Autodesk Fusion 360 part; units mm, degrees
sketch "Skizze1" plane through (0, 0, 0) normal (0, 0, 1) x (1, 0, 0)
  line L0 (0, 0) -> (60, 0)
  line L1 (60, 0) -> (60, 140)
  line L2 (60, 140) -> (0, 140)
  line L3 (0, 140) -> (0, 0)
  dimension "d1" = 60
  dimension "d2" = 140
extrude "Extrusion1" add sketch "Skizze1" along normal blind 20
sketch "Skizze2" plane through (60, 0, 0) normal (1, 0, 0) x (0, 1, 0)
  line L0 (0, 0) -> (140, 0)
  line L1 (140, 0) -> (140, 20)
  line L2 (140, 20) -> (0, 20)
  line L3 (0, 20) -> (0, 0)
  circle A0 centre (30, 10) radius 4.15
  circle A1 centre (100.3, 10) radius 4.15
  point P0 (0, 10)
  dimension "d5" = 8.3
  dimension "d6" = 8.3
extrude "Extrusion2" cut sketch "Skizze2" against normal blind 50 contours A0 | A1
sketch "Skizze3" plane through (0, 0, 20) normal (0, 0, 1) x (-1, 0, 0)
  line L0 (0, -140) -> (0, 0)
  line L1 (0, 0) -> (-60, 0)
  line L2 (-60, 0) -> (-60, -140)
  line L3 (-60, -140) -> (0, -140)
  circle A0 centre (-31.6, -24.1) radius 1.7
  circle A1 centre (-7.7, -24.1) radius 1.7
  circle A2 centre (-31.6, -6.2) radius 1.7
  circle A3 centre (-7.7, -6.2) radius 1.7
  circle A4 centre (-7.7, -107.4) radius 1.7
  circle A5 centre (-31.6, -125.3) radius 1.7
  circle A6 centre (-7.7, -125.3) radius 1.7
  circle A7 centre (-31.6, -107.4) radius 1.7
  dimension "d9" = 3.4
  dimension "d10" = 3.4
  dimension "d11" = 3.4
  dimension "d12" = 3.4
  dimension "d13" = 3.4
  dimension "d14" = 3.4
  dimension "d15" = 3.4
  dimension "d16" = 3.4
extrude "Extrusion3" cut sketch "Skizze3" against normal blind 20 contours A0 | A1 | A2 | A3 | A4 | A5 | A6 | A7
sketch "Skizze5" plane through (0, 0, 0) normal (0, 0, -1) x (1, 0, 0)
  line L0 (0, 0) -> (0, -140)
  line L1 (0, -140) -> (60, -140)
  line L2 (60, -140) -> (60, 0)
  line L3 (60, 0) -> (0, 0)
  circle A0 centre (46, -130) radius 1
  circle A1 centre (7.7, -125.3) radius 1.7
  circle A2 centre (31.6, -24.1) radius 1.7
  circle A3 centre (31.6, -6.2) radius 1.7
  circle A4 centre (31.6, -125.3) radius 1.7
  circle A5 centre (7.7, -107.4) radius 1.7
  circle A6 centre (7.7, -24.1) radius 1.7
  circle A7 centre (7.7, -6.2) radius 1.7
  circle A8 centre (31.6, -107.4) radius 1.7
  dimension "d22" = 2
sketch "Skizze6" plane through (0, 0, 0) normal (0, 0, -1) x (1, 0, 0)
  circle A0 centre (7.7, -125.3) radius 1.7
  circle A1 centre (31.6, -24.1) radius 1.7
  circle A2 centre (31.6, -6.2) radius 1.7
  circle A3 centre (31.6, -125.3) radius 1.7
  circle A4 centre (7.7, -107.4) radius 1.7
  circle A5 centre (7.7, -24.1) radius 1.7
  circle A6 centre (7.7, -6.2) radius 1.7
  circle A7 centre (31.6, -107.4) radius 1.7
  line L0 (0, 0) -> (0, -140)
  line L1 (0, -140) -> (60, -140)
  line L2 (60, -140) -> (60, 0)
  line L3 (60, 0) -> (0, 0)
  line L4 (60, -53.1468) -> (40, -53.1468)
  line L5 (40, -53.1468) -> (40, -85.1468)
  line L6 (40, -85.1468) -> (60, -85.1468)
  line L7 (60, -85.1468) -> (60, -53.1468)
  line L8 (60, -53.1468) -> (40, -53.1468)
  line L9 (40, -53.1468) -> (40, -58.1468)
  line L10 (40, -58.1468) -> (60, -58.1468)
  line L11 (60, -58.1468) -> (60, -53.1468)
  line L12 (40, -85.1468) -> (60, -85.1468)
  line L13 (60, -85.1468) -> (60, -80.1468)
  line L14 (60, -80.1468) -> (40, -80.1468)
  line L15 (40, -80.1468) -> (40, -85.1468)
  line L16 (53.5, -63.5) -> (36.5, -63.5)
  arc A8 (36.5, -63.5) -> (36.5, -66.5) centre (36.5, -65) ccw
  line L17 (36.5, -66.5) -> (53.5, -66.5)
  arc A9 (53.5, -66.5) -> (53.5, -63.5) centre (53.5, -65) ccw
  line L18 (55, -65) -> (35, -65) construction
  line L19 (36.5, -75.4708) -> (53.5, -75.4708)
  arc A10 (53.5, -75.4708) -> (53.5, -72.4708) centre (53.5, -73.9708) ccw
  line L20 (53.5, -72.4708) -> (36.5, -72.4708)
  arc A11 (36.5, -72.4708) -> (36.5, -75.4708) centre (36.5, -73.9708) ccw
  line L21 (35, -73.9708) -> (55, -73.9708) construction
  dimension "d31" = 20
  dimension "d32" = 32
  dimension "d33" = 20
  dimension "d34" = 5
  dimension "d35" = 20
  dimension "d36" = 5
  dimension "d72" = 3
  dimension "d73" = 3
extrude "Extrusion19" cut sketch "Skizze6" against normal blind 1 contours L5 L16 L17 A9 | L5 L16 A8 L17 | L5 L19 L20 A11 | L5 L19 A10 L20
extrude "Extrusion7" add sketch "Skizze6" along normal blind 12 contours L2 L4 L5 L7 L8 L9 L10 L11 | L2 L5 L6 L7 L12 L13 L14 L15
sketch "Skizze8" plane through (0, 0, 0) normal (-1, 0, 0) x (0, -1, 0)
  line L0 (-140, 0) -> (0, 0)
  line L1 (0, 0) -> (0, 20)
  line L2 (0, 20) -> (-140, 20)
  line L3 (-140, 20) -> (-140, 0)
  circle A0 centre (-15, 10) radius 2.2
  circle A1 centre (-45, 10) radius 2.2
  dimension "d27" = 4.4
  dimension "d28" = 4.4
extrude "Extrusion6" cut sketch "Skizze8" against normal blind 60 contours A0 | A1
sketch "Skizze10" plane through (60, 0, 0) normal (1, 0, 0) x (0, 1, 0)
  line L0 (58.1468, -12) -> (58.1468, 0)
  line L1 (58.1468, 0) -> (80.1468, 0)
  line L2 (80.1468, 0) -> (80.1468, -12)
  circle A0 centre (15, 10) radius 2.2
  circle A1 centre (45, 10) radius 2.2
  circle A2 centre (30, 10) radius 4.15
  circle A3 centre (100.3, 10) radius 4.15
  line L3 (53.1468, -12) -> (58.1468, -12)
  line L4 (85.1468, -12) -> (85.1468, 0)
  line L5 (85.1468, 0) -> (140, 0)
  line L6 (140, 0) -> (140, 20)
  line L7 (140, 20) -> (0, 20)
  line L8 (0, 20) -> (0, 0)
  line L9 (0, 0) -> (53.1468, 0)
  line L10 (53.1468, 0) -> (53.1468, -12)
  circle A4 centre (15, 10) radius 7.5
  circle A5 centre (45, 10) radius 7.5
  line L11 (80.1468, -12) -> (85.1468, -12)
  dimension "d42" = 15
  dimension "d43" = 15
extrude "Extrusion9" cut sketch "Skizze10" against normal blind 10 contours A4 | A5
sketch "Skizze13" plane through (0, 0, 20) normal (0, 0, 1) x (-1, 0, 0)
  circle A0 centre (-7.7, -125.3) radius 1.7
  circle A1 centre (-31.6, -24.1) radius 1.7
  circle A2 centre (-31.6, -6.2) radius 1.7
  circle A3 centre (-31.6, -125.3) radius 1.7
  circle A4 centre (-7.7, -107.4) radius 1.7
  circle A5 centre (-7.7, -24.1) radius 1.7
  circle A6 centre (-7.7, -6.2) radius 1.7
  circle A7 centre (-31.6, -107.4) radius 1.7
  line L0 (0, -140) -> (0, 0)
  line L1 (0, 0) -> (-60, 0)
  line L2 (-60, 0) -> (-60, -140)
  line L3 (-60, -140) -> (0, -140)
  circle A8 centre (-47, -10) radius 7.5
  dimension "d53" = 15
extrude "Extrusion12" cut sketch "Skizze13" against normal blind 5 contours A8
sketch "Skizze14" plane through (0, 0, 15) normal (0, 0, 1) x (-1, 0, 0)
  line L0 (-50, -9.4098) -> (-50, -16.8739)
  arc A0 (-50, -16.8739) -> (-54.4767, -9.4098) centre (-47, -10) ccw
  line L1 (-54.4767, -9.4098) -> (-50, -9.4098)
  circle A1 centre (-47, -10) radius 1
  dimension "d56" = 2
extrude "Extrusion13" cut sketch "Skizze14" against normal blind 1 contours A1
sketch "Skizze15" plane through (0, 0, 20) normal (0, 0, 1) x (-1, 0, 0)
  circle A0 centre (-47, -10) radius 7.5
  circle A1 centre (-7.7, -125.3) radius 1.7
  circle A2 centre (-31.6, -24.1) radius 1.7
  circle A3 centre (-31.6, -6.2) radius 1.7
  circle A4 centre (-31.6, -125.3) radius 1.7
  circle A5 centre (-7.7, -107.4) radius 1.7
  circle A6 centre (-7.7, -24.1) radius 1.7
  circle A7 centre (-7.7, -6.2) radius 1.7
  circle A8 centre (-31.6, -107.4) radius 1.7
  line L0 (0, -140) -> (0, 0)
  line L1 (0, 0) -> (-60, 0)
  line L2 (-60, 0) -> (-60, -140)
  line L3 (-60, -140) -> (0, -140)
  line L4 (-39.5, 0) -> (-54.5, 0)
  line L5 (-54.5, 0) -> (-54.5, -17.5)
  line L6 (-54.5, -17.5) -> (-39.5, -17.5)
  line L7 (-39.5, -17.5) -> (-39.5, 0)
extrude "Extrusion14" cut sketch "Skizze15" against normal blind 7 contours A0 | A0 L1 L4 L5 L7
sketch "Skizze16" plane through (0, 0, 20) normal (0, 0, 1) x (-1, 0, 0)
  circle A0 centre (-31.6, -107.4) radius 1.7
  circle A1 centre (-7.7, -6.2) radius 1.7
  circle A2 centre (-7.7, -24.1) radius 1.7
  circle A3 centre (-7.7, -107.4) radius 1.7
  circle A4 centre (-31.6, -125.3) radius 1.7
  circle A5 centre (-31.6, -6.2) radius 1.7
  circle A6 centre (-31.6, -24.1) radius 1.7
  circle A7 centre (-7.7, -125.3) radius 1.7
  line L0 (-39.5, 0) -> (-39.5, -10)
  arc A8 (-54.5, -10) -> (-39.5, -10) centre (-47, -10) ccw
  line L1 (-54.5, -10) -> (-54.5, 0)
  line L2 (-54.5, 0) -> (-60, 0)
  line L3 (-60, 0) -> (-60, -140)
  line L4 (-60, -140) -> (0, -140)
  line L5 (0, -140) -> (0, 0)
  line L6 (0, 0) -> (-39.5, 0)
  circle A9 centre (-46, -130) radius 7.5
  line L7 (-38.5, -140) -> (-53.5, -140)
  line L8 (-53.5, -140) -> (-53.5, -122.5)
  line L9 (-53.5, -122.5) -> (-38.5, -122.5)
  line L10 (-38.5, -122.5) -> (-38.5, -140)
  dimension "d61" = 15
extrude "Extrusion15" cut sketch "Skizze16" against normal blind 7 contours L4 A9 L7 L8 L10 | A9
sketch "Skizze17" plane through (0, 0, 20) normal (0, 0, 1) x (-1, 0, 0)
  line L0 (-38.5, -130) -> (-38.5, -140)
  line L1 (-38.5, -140) -> (0, -140)
  line L2 (0, -140) -> (0, 0)
  line L3 (0, 0) -> (-39.5, 0)
  line L4 (-39.5, 0) -> (-39.5, -10)
  arc A0 (-54.5, -10) -> (-39.5, -10) centre (-47, -10) ccw
  line L5 (-54.5, -10) -> (-54.5, 0)
  line L6 (-54.5, 0) -> (-60, 0)
  line L7 (-60, 0) -> (-60, -140)
  line L8 (-60, -140) -> (-53.5, -140)
  line L9 (-53.5, -140) -> (-53.5, -130)
  arc A1 (-38.5, -130) -> (-53.5, -130) centre (-46, -130) ccw
  circle A2 centre (-31.6, -107.4) radius 1.7
  circle A3 centre (-7.7, -6.2) radius 1.7
  circle A4 centre (-7.7, -24.1) radius 1.7
  circle A5 centre (-7.7, -107.4) radius 1.7
  circle A6 centre (-31.6, -125.3) radius 1.7
  circle A7 centre (-31.6, -6.2) radius 1.7
  circle A8 centre (-31.6, -24.1) radius 1.7
  circle A9 centre (-7.7, -125.3) radius 1.7
  line L10 (-49.25, -92.5) -> (-42.75, -92.5)
  line L11 (-42.75, -92.5) -> (-42.75, -152.5)
  line L12 (-42.75, -152.5) -> (-49.25, -152.5)
  line L13 (-49.25, -152.5) -> (-49.25, -92.5)
  line L14 (-49.25, -92.5) -> (-42.75, -152.5) construction
  line L15 (-42.75, -92.5) -> (-49.25, -152.5) construction
  point P0 (-46, -122.5)
  dimension "d64" = 60
  dimension "d65" = 6.5
extrude "Extrusion16" cut sketch "Skizze17" against normal blind 5 contours A1 L10 L11 L13
sketch "Skizze18" plane through (0, 0, 20) normal (0, 0, 1) x (-1, 0, 0)
  line L0 (-42.75, -92.5) -> (-42.75, -123.2407)
  arc A0 (-38.5, -130) -> (-42.75, -123.2407) centre (-46, -130) ccw
  line L1 (-38.5, -130) -> (-38.5, -140)
  line L2 (-38.5, -140) -> (0, -140)
  line L3 (0, -140) -> (0, 0)
  line L4 (0, 0) -> (-39.5, 0)
  line L5 (-39.5, 0) -> (-39.5, -10)
  arc A1 (-54.5, -10) -> (-39.5, -10) centre (-47, -10) ccw
  line L6 (-54.5, -10) -> (-54.5, 0)
  line L7 (-54.5, 0) -> (-60, 0)
  line L8 (-60, 0) -> (-60, -140)
  line L9 (-60, -140) -> (-53.5, -140)
  line L10 (-53.5, -140) -> (-53.5, -130)
  arc A2 (-49.25, -123.2407) -> (-53.5, -130) centre (-46, -130) ccw
  line L11 (-49.25, -123.2407) -> (-49.25, -92.5)
  line L12 (-49.25, -92.5) -> (-42.75, -92.5)
  circle A3 centre (-31.6, -107.4) radius 1.7
  circle A4 centre (-7.7, -6.2) radius 1.7
  circle A5 centre (-7.7, -24.1) radius 1.7
  circle A6 centre (-7.7, -107.4) radius 1.7
  circle A7 centre (-31.6, -125.3) radius 1.7
  circle A8 centre (-31.6, -6.2) radius 1.7
  circle A9 centre (-31.6, -24.1) radius 1.7
  circle A10 centre (-7.7, -125.3) radius 1.7
  line L13 (-50.25, -47.5) -> (-43.75, -47.5)
  line L14 (-43.75, -47.5) -> (-43.75, 12.5)
  line L15 (-43.75, 12.5) -> (-50.25, 12.5)
  line L16 (-50.25, 12.5) -> (-50.25, -47.5)
  line L17 (-50.25, -47.5) -> (-43.75, 12.5) construction
  line L18 (-43.75, -47.5) -> (-50.25, 12.5) construction
  point P0 (-47, -17.5)
  dimension "d68" = 6.5
  dimension "d69" = 60
extrude "Extrusion17" cut sketch "Skizze18" against normal blind 5 contours A1 L13 L14 L16
extrude "Extrusion18" cut 2 faces at (46.6667, 54.8135, -12) (53.3333, 83.4802, -12) along direction (0, 0, 1) blind 12
CAD build for the part. Positions are in the model's coordinates, mm. A direction names the side the tool comes from. Coordinates: 2 decimals unless noted, no trailing zeros. Write each loop counter-clockwise with the first axis right and the second up, starting at its lowest first coordinate (ties: lowest second). Pieces come first, ordered by that corner, then holes.
(1) Cut at B-B, the plane y = 6.2. List the corners of the cut face in (x, z).
(2) Cut at A-A, the plane x = 31.6. Count the separate pieces of the cut face and the enclosed holes in it, and give its area (3 significant figures).
(3) Cut at C-C, the plane x = 19. List the corners of the cut face in (y, z).
(4) Drill centre lines: probe 1 along Y at (x, z) = (31.6, 15); probe 2 along Y at (x, z) = (47, 10.5); probe 3 along Z at (x, y) = (48, 30). Where is each one in solid material? Low to high.
(5) Two-plate mould, pull along Y, no slides. Class faces 6 (the face through (38.5, 135, 17)), 7 (the face through (50, 47, 8)), 8 (the face through (41.693, 15.3, 15.771)), 9 (the face through (10, 30, 10)): +Y half, -Y half, draft (parallel to the pull), parting line (faces both ways), or undercut.
(6) 3-axis set-ups, long thin cutter, end or side, ignore diameter. For faces 1 (the face through (54.5, 5, 17)), 2 (the face through (10, 100, 10)), 3 (the face through (30.8, 25.6, 10.1)), 4 (the face through (53.5, 135, 17)), 5 (the face through (45, 65, 1)): which of +Z, -Z, +X, -X, +Y, -Y reach the whole face in a straight line?
(7) Flat gauge pins, fed straight in: pin 1 (4 mm diameter, centred on x = 46, z = 17.5, fed in from -Y); pin 2 (7.5 mm diameter, centred on x = 43.5, y = 129, fed in from +Z). Where does each tip first touch, or does it go through?
Geometry says:
1. outline: (0, 0) - (6, 0) - (6, 20) - (0, 20) - close; (9.4, 0) - (29.9, 0) - (29.9, 20) - (9.4, 20) - close; (33.3, 0) - (60, 0) - (60, 20) - (54.5, 20) - (54.5, 13) - (39.5, 13) - (39.5, 20) - (33.3, 20) - close
2. separate pieces: 5
2. enclosed holes: 4
2. area: 2,390 mm2
3. outline: (0, 0) - (140, 0) - (140, 20) - (0, 20) - close; hole circle Ø4.4 at (15, 10); hole circle Ø8.3 at (30, 10); hole circle Ø4.4 at (45, 10); hole circle Ø8.3 at (100.3, 10)
4. probe 1: y = 0 to 4.5, 7.9 to 22.4, 25.8 to 105.7, 109.1 to 123.6, 127 to 140
4. probe 2: y = 0 to 12.86, 17.14 to 25.88, 34.12 to 42.86, 47.14 to 96.18, 104.42 to 140
4. probe 3: z = 0 to 5.85, 14.15 to 15
5. face 6: draft
5. face 7: undercut
5. face 8: -Y half
5. face 9: undercut
6. face 1: +Z, -Y
6. face 2: +X
6. face 3: +Z, -Z
6. face 4: +Z, +Y
6. face 5: -Z
7. pin 1: stops at y = 47.5
7. pin 2: stops at z = 13
